```python
from build123d import *

# Parameters (mm, degrees)
F2_W     = 5.528318
F2_H     = 2.70489
F3_DEPTH = 4.318
F4_R     = 1.27
F5_DEPTH = 3.176


with BuildPart() as f1:
    # F0 (on Front) → F1 (revolve)
    with BuildSketch(Plane.XZ):
        Polygon((6.35, 13.462), (0, 13.462), (0, 10.922), (4.7625, 10.922), (4.7625, 0), (12.7, 0), (12.7, 3.175), (6.35, 3.175), align=None)
    revolve(axis=Axis((0, 0, 12.192), (0, 0, 1)))

    # F2 (on face) → F3 (join)
    with BuildSketch(Plane.XY.offset(13.462)):
        Rectangle(F2_W, F2_H)
    extrude(amount=F3_DEPTH)

    # F4 (on face) → F5 (cut, through all)
    with BuildSketch(Plane.XY.offset(3.175)):
        with Locations((-9.525, 0)):
            Circle(F4_R)
        with Locations((9.525, 0)):
            Circle(F4_R)
    extrude(amount=-F5_DEPTH, mode=Mode.SUBTRACT)


solid = f1.part
```
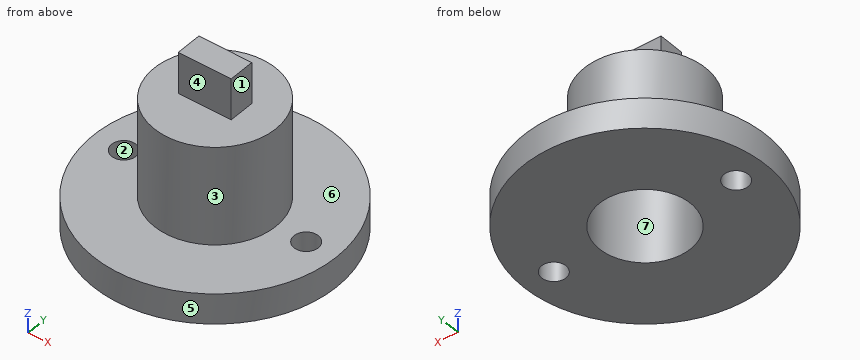
CAD build for the part. Positions are in the model's coordinates, mm. Face numbers are marked on the shaded views. A direction names the side the tool comes from. Round coordinates to 2 decimals unless told otherwise and drop trailing zeros. Order: outer loops, then holes, each group sorted by start corner. A loop starts at its lowest first (then second) coordinate and runs counter-clockwise, first axis right, second up.
Item 1: Saw through at D-D on y = 4. Write the cut outline in (x, z) (3 decimals).
Item 2: Pin check, flat tips, straight feed: pin 1 (1.3 mm diameter, centred on x = 1, z = 15.5, fed in from -Y); pin 2 (3 mm diameter, centred on y = 3, z = 7, fed in from +X); pin 3 (0.8 mm diameter, centred on y = 0, z = 16, fed in from -X); pin 4 (2 mm diameter, centred on x = 9.525, y = 0, fed in from -Z). Stop position of each tip, or through.
Item 3: Saw through at C-C on z = 1.5. Write the cut outline in (x, y) (1 decimal).
Item 4: Mould opens along Y. For the marked faces 1, 2 and 3 say: pulls with the +Y half, pulls with the -Y half, needs draft (parallel to the pull), parting line crosses it, or undercut.
Item 5: Probe line 1 along Z through (x, y) = (-3.25, -1.5); line 2 along Y through (x, z) = (0, 8); line 3 along Z through (x, y) = (7.75, -1.5) (3 decimals). List the from-to ranges inside material, lowest first.
Item 6: Tool access for the marked faces 4, 5, 6 and 7: list every direction of +Z, -Z, +X, -X, +Y, -Y with a clear straight run to the whole face (end or side of a thin tool).
Item 7: Saw through at A-A on y = 0. State how many separate pieces and enclosed holes the cut face has, then the cut area to 3 significant figures.
Reported:
1. outline: (-12.054, 0) - (-2.585, 0) - (-2.585, 10.922) - (2.585, 10.922) - (2.585, 0) - (12.054, 0) - (12.054, 3.175) - (4.932, 3.175) - (4.932, 13.462) - (-4.932, 13.462) - (-4.932, 3.175) - (-12.054, 3.175) - close
2. pin 1: stops at y = -1.35
2. pin 2: stops at x = 6.17
2. pin 3: stops at x = -2.76
2. pin 4: passes through
3. outline: circle Ø25.4 at (0, 0); hole circle Ø2.5 at (-9.5, 0); hole circle Ø9.5 at (0, 0); hole circle Ø2.5 at (9.5, 0)
4. face 1: needs draft
4. face 2: undercut
4. face 3: parting line crosses it
5. line 1: z = 10.92 to 13.46
5. line 2: y = -6.35 to -4.76, 4.76 to 6.35
5. line 3: z = 0 to 3.175
6. face 4: +Z, +X, -X, -Y
6. face 5: +Z, -Z
6. face 6: +Z
6. face 7: -Z
7. separate pieces: 3
7. enclosed holes: 0
7. area: 115 mm2
